Input: dimensioned drawing with shaded views. Units: mm. Origin: part minimum x, y, z. Round coordinates to 2 decimals unless told otherwise and drop trailing zeros. Loops run counter-clockwise (first coordinate to the right, second up) from the corner with the lowest first, then second, coordinate; pieces in that order, holes last.
1) Section C-C, the plane z = 2.35. Return loops of the section in (x, y), and give its area (3 significant figures).
2) First-contact query: pin 1 (1 mm diameter, centred on y = 23.5, z = 4.5, fed in from -X); pin 2 (3 mm diameter, centred on x = 59.5, y = 11, fed in from +Z); pin 3 (2.5 mm diameter, centred on y = 30, z = 3.5, fed in from +X). Flat tips, straight axial feed; report the tip coordinate or a pass-through.
3) Section B-B, the plane x = 55. Return loops of the section in (y, z).
4) Section A-A, the plane y = 23.5. Return loops of the section in (x, z), and give its area (3 significant figures).
5) Ray query, line 1 along Y through (x, z) = (38, 1.6); line 2 along X through (y, z) = (14, 0.9); line 3 along X through (y, z) = (23.5, 4.1). Return the intervals inside material, ascending.
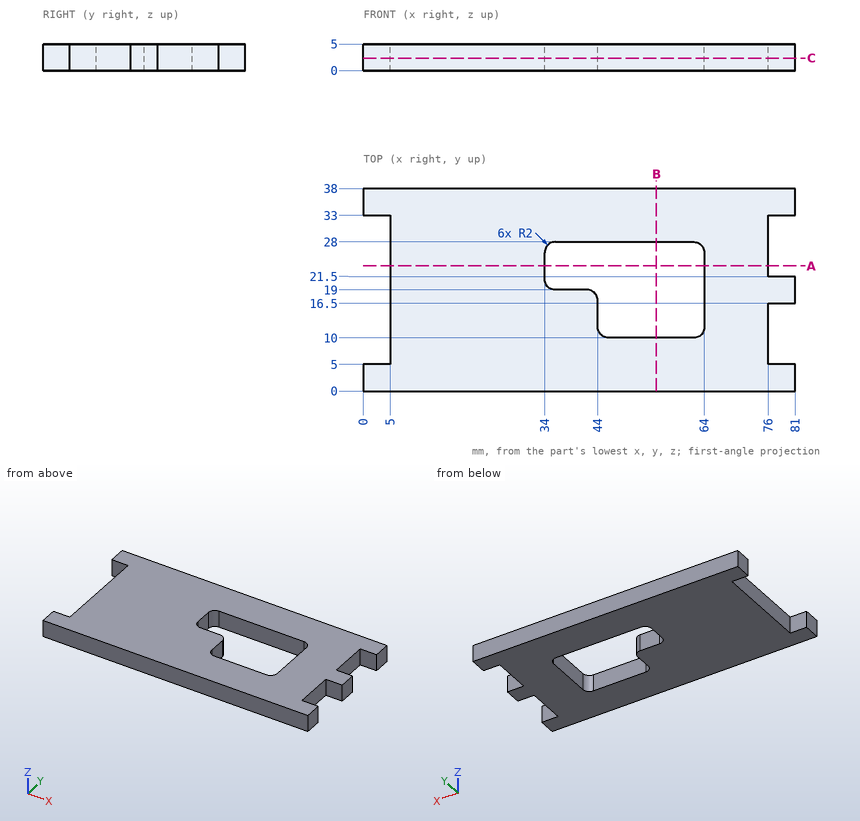
Final values:
1. outline: (0, 0) - (81, 0) - (81, 5) - (76, 5) - (76, 16.5) - (81, 16.5) - (81, 21.5) - (76, 21.5) - (76, 33) - (81, 33) - (81, 38) - (0, 38) - (0, 33) - (5, 33) - (5, 5) - (0, 5) - close; hole (34, 21) arc R2 ccw to (36, 19) - (42, 19) arc R2 cw to (44, 17) - (44, 12) arc R2 ccw to (46, 10) - (62, 10) arc R2 ccw to (64, 12) - (64, 26) arc R2 ccw to (62, 28) - (36, 28) arc R2 ccw to (34, 26) - close
1. area: 2,380 mm2
2. pin 1: stops at x = 5
2. pin 2: stops at z = 5
2. pin 3: stops at x = 76
3. outline: (0, 0) - (10, 0) - (10, 5) - (0, 5) - close; (28, 0) - (38, 0) - (38, 5) - (28, 5) - close
4. outline: (5, 0) - (34, 0) - (34, 5) - (5, 5) - close; (64, 0) - (76, 0) - (76, 5) - (64, 5) - close
4. area: 205 mm2
5. line 1: y = 0 to 19, 28 to 38
5. line 2: x = 5 to 44, 64 to 76
5. line 3: x = 5 to 34, 64 to 76
